```python
from build123d import *

# Parameters (mm, degrees)
SKETCH1_R           = 36.83
BOSS_EXTRUDE1_DEPTH = 17.78
FILLET1_R           = 2.54
SKETCH2_R           = 26.67
SKETCH3_R           = 14.7955
SKETCH4_R           = 14.7955
CUT_EXTRUDE1_DEPTH  = 76.2
SKETCH7_R           = 14.7955
SKETCH6_R           = 36.83
SKETCH8_R           = 31.75
SKETCH8_R_2         = 29.21
CUT_EXTRUDE2_DEPTH  = 2.54
FILLET3_R           = 2.54
FILLET4_R           = 2.54
FILLET5_R           = 2.54


with BuildPart() as part:
    # Sketch1 → Boss-Extrude1 (new body)
    with BuildSketch(Plane(origin=(0, 0, 0), x_dir=(1, 0, 0), z_dir=(0, 1, 0))):
        with Locations(Location((0, 0, 0), (0, 0, 90))):
            Circle(SKETCH1_R)
    extrude(amount=BOSS_EXTRUDE1_DEPTH)

    # Fillet1
    fillet1_edges = [part.edges().sort_by_distance(p)[0] for p in [
        (0, 0, 36.83),
    ]]
    fillet(fillet1_edges, radius=FILLET1_R)

    # Sketch2 → Cut-Loft1 section 0
    with BuildSketch(Plane(origin=(0, 0, 0), x_dir=(1, 0, 0), z_dir=(0, 1, 0))):
        Circle(SKETCH2_R)
    # Sketch3 → Cut-Loft1 section 1
    with BuildSketch(Plane(origin=(0, 11.938, 0), x_dir=(1, 0, 0), z_dir=(0, 1, 0))):
        Circle(SKETCH3_R)
    loft(mode=Mode.SUBTRACT)

    # Sketch4 → Cut-Extrude1 (cut)
    with BuildSketch(Plane.XZ.offset(-11.938)):
        with Locations(Location((0, 0, 0), (0, 0, 270))):
            Circle(SKETCH4_R)
    extrude(amount=-CUT_EXTRUDE1_DEPTH, mode=Mode.SUBTRACT)

    # Sketch7 → Cut-Loft2 section 0
    with BuildSketch(Plane(origin=(0, 11.43, 0), x_dir=(1, 0, 0), z_dir=(0, 1, 0))):
        Circle(SKETCH7_R)
    # Sketch6 → Cut-Loft2 section 1
    with BuildSketch(Plane(origin=(0, 17.78, 0), x_dir=(1, 0, 0), z_dir=(0, 1, 0))):
        Circle(SKETCH6_R)
    loft(mode=Mode.SUBTRACT)

    # Sketch8 → Cut-Extrude2 (cut)
    with BuildSketch(Plane.XZ):
        with Locations(Location((0, 0, 0), (0, 0, 270))):
            Circle(SKETCH8_R)
        with Locations(Location((0, 0, 0), (0, 0, 270))):
            Circle(SKETCH8_R_2, mode=Mode.SUBTRACT)
    extrude(amount=-CUT_EXTRUDE2_DEPTH, mode=Mode.SUBTRACT)

    # Fillet3
    fillet3_edges = [part.edges().sort_by_distance(p)[0] for p in [
        (0, 0, 31.75),
    ]]
    fillet(fillet3_edges, radius=FILLET3_R - 0.0001)  # a hair under: the kernel refuses the full size

    # Fillet4
    fillet4_edges = [part.edges().sort_by_distance(p)[0] for p in [
        (0, 0, 29.21),
    ]]
    fillet(fillet4_edges, radius=FILLET4_R - 0.0001)  # a hair under: the kernel refuses the full size

    # Fillet5
    fillet5_edges = [part.edges().sort_by_distance(p)[0] for p in [
        (-15.18822317, 11.543176706, 0),
    ]]
    fillet(fillet5_edges, radius=FILLET5_R)


solid = part.part
```
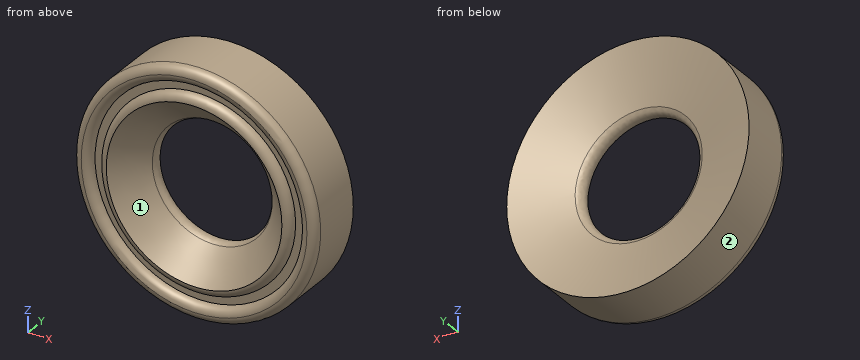
Input: part model. Units: mm. Frame: model coordinates. Face numbers are marked on the shaded views. Give positions to 0.01 mm unless a question says otherwise; leave off trailing zeros. Order: outer loops, then holes, each group sorted by start corner. A loop starts at its lowest first (then second) coordinate and runs counter-clockwise, first axis right, second up. Notation, with made-up numbers: M 78.25,-39.75 L 133.25,-39.75 A28 ccw 133.25,-12.75 Z; hole C -2,-17 d4. An arc over 180 degrees is marked long. One line per question, with ' | ' between items. Start each with the question number.
1. Material intervals for probe 1 along Z at (x, y) = (21, 2.5); probe 2 along X at (y, z) = (2, 25); probe 3 along X at (y, z) = (2.5, 0), sorted ascending. Write a range as [from, to].
2. Pull-direction query (X, two-part tool) for the marked faces 1 and 2; classes: released by +X, released by -X, zero draft, split by the parting line, or undercut.
3. Section query C-C (y = 14.25). Return the cut outline in (x, z).
4. First-contact query: pin 1 Ø4 at (x, y) = (16.5, 2.5) entering from +Z; pin 2 Ø4 at (x, y) = (-8, 8) entering from +Z; pin 3 Ø10 at (y, z) = (11.5, -29) entering from -X. Flat tips, straight axial feed; report the tip coordinate or a pass-through.
5. Section query A-A (y = 1.5). Return the cut outline in (x, z).
6. Section query B-B (y = 7.25). Return the cut outline in (x, z).
Here are the results:
1) probe 1: [-30.26, -23.81], [-20.3, -11.99], [11.99, 20.3], [23.81, 30.26] | probe 2: [-26.97, -19.67], [-14.99, 14.99], [19.67, 26.97] | probe 3: [-36.83, -31.75], [-29.21, -24.18], [24.18, 29.21], [31.75, 36.83]
2) face 1: undercut | face 2: split by the parting line
3) outline: C 0,0 d73.66; hole C 0,0 d49.16
4) pin 1: z = 33.86 | pin 2: z = 36.34 | pin 3: x = -27.94
5) outline: C 0,0 d73.21; C 0,0 d57.97; hole C 0,0 d63.95; hole C 0,0 d50.36
6) outline: C 0,0 d73.66; hole C 0,0 d38.92
